Geometry check sheet. Reference: the model listing, model coordinates, mm. A direction names the side the tool comes from. Coordinates: 2 decimals unless noted, no trailing zeros. Loops run counter-clockwise (first coordinate to the right, second up) from the corner with the lowest first, then second, coordinate; pieces in that order, holes last. Notation, with made-up numbers: M -17,49.25 L 16,49.25 A25 cw 16,84.25 Z; hole C 52,67 d2. An arc over 180 degrees is marked long. Use CSV: the item, a comma, the result in double quotes.
```python
from build123d import *

# Parameters (mm, degrees)
EXTRUDE004_DEPTH                     = 10
SKETCH008_R                          = 3.1
EXTRUDE003_DEPTH                     = 10
EXTRUDE002_DEPTH                     = 2.65
EXTRUDE002_ONTO_SKETCH004_ROLL_ANGLE = 90
EXTRUDE001_DEPTH                     = 14
EXTRUDE_DEPTH                        = 30
EXTRUDE_ONTO_SKETCH_ROLL_ANGLE       = 90
FILLET_R                             = 10
POCKET_DEPTH                         = 20.001
SKETCH003_R                          = 1.55
POCKET001_DEPTH                      = 8
SKETCH005_W                          = 6
SKETCH005_H                          = 4
POCKET002_DEPTH                      = 9.5
SKETCH006_R                          = 4.1
POCKET003_DEPTH                      = 14.35
FILLET001_R                          = 2.5
FILLET002_R                          = 1
FILLET003_R                          = 2.5
FILLET004_R                          = 0.95
CHAMFER_SIZE2                        = 16
CHAMFER_SIZE                         = 6
CHAMFER001_SIZE                      = 5
SKETCH007_R                          = 1.55
POCKET004_DEPTH                      = 5.726
POCKET004_DEPTH_BACK                 = 6.476
FILLET005_R                          = 5
FILLET006_R                          = 0.65


with BuildPart() as extrude004:
    # Sketch009 → Extrude004 (new body)
    with BuildSketch(Plane(origin=(0.375, 0, 0), x_dir=(0, -1, 0), z_dir=(-1, 0, 0))):
        Polygon((-21.182001, 11.641407), (-23.86668, 10.091407), (-23.86668, 6.991407), (-21.182001, 5.441407), (-18.497322, 6.991407), (-18.497322, 10.091407), align=None)
    extrude(amount=-EXTRUDE004_DEPTH)


with BuildPart() as extrude004_1:
    # Extrude004 placement: moved
    add(extrude004.part.moved(Location((2, 0, 0))))


with BuildPart() as extrude003:
    # Sketch008 → Extrude003 (new body)
    with BuildSketch(Plane.YZ.offset(-0.375)):
        with Locations((21.182001, 8.541407)):
            Circle(SKETCH008_R)
    extrude(amount=-EXTRUDE003_DEPTH)


with BuildPart() as extrude003_1:
    # Extrude003 placement: moved
    add(extrude003.part.moved(Location((-2, 0, 0))))


with BuildPart() as extrude002:
    # Sketch004 as drawn → Extrude002 (new)
    with BuildSketch(Plane.XY):
        Polygon((0, -0.237971), (-2.825, -1.868985), (-2.825, -7), (2.825, -7), (2.825, -1.868985), align=None)
    extrude(amount=-EXTRUDE002_DEPTH)


with BuildPart() as extrude002_1:
    # Extrude002 onto Sketch004 roll: moved
    add(extrude002.part.rotate(Axis((0, 0, 0), (1, 0, 0)), EXTRUDE002_ONTO_SKETCH004_ROLL_ANGLE))


with BuildPart() as extrude002_2:
    # Extrude002 onto Sketch004 placement: moved
    add(extrude002_1.part.moved(Location((0, 4, 0))))


with BuildPart() as extrude002_3:
    # Extrude002 placement: moved
    add(extrude002_2.part.moved(Location((0, 3, 0))))


with BuildPart() as extrude001:
    # Sketch001 → Extrude001 (new body)
    with BuildSketch(Plane.YZ):
        Polygon((0, -7), (0, 0), (4, -3.5), (4, -7), align=None)
    extrude(amount=EXTRUDE001_DEPTH)


with BuildPart() as extrude001_1:
    # Extrude001 placement: moved
    add(extrude001.part.moved(Location((-7, 0, 0))))


with BuildPart() as fillet006:
    # Sketch as drawn → Extrude (new)
    with BuildSketch(Plane.XY):
        with BuildLine():
            Line((-6.1, -7), (6.1, -7))
            Line((6.1, -7), (6.1, 3.217039))
            Line((6.1, 3.217039), (4.375, 13))
            Line((4.375, 13), (0.375, 13))
            Line((0.375, 13), (0.375, 0.927025))
            ThreePointArc((-0.375, 0.927025), (0, -1), (0.375, 0.927025))
            Line((-0.375, 0.927025), (-0.375, 13))
            Line((-0.375, 13), (-4.375, 13))
            Line((-4.375, 13), (-6.1, 3.217039))
            Line((-6.1, 3.217039), (-6.1, -7))
        make_face()
    extrude(amount=-EXTRUDE_DEPTH)


with BuildPart() as fillet006_1:
    # Extrude onto Sketch roll: moved
    add(fillet006.part.rotate(Axis((0, 0, 0), (1, 0, 0)), EXTRUDE_ONTO_SKETCH_ROLL_ANGLE))


with BuildPart() as fillet006_2:
    # Extrude onto Sketch placement: moved
    add(fillet006_1.part)

    # Fillet
    fillet_edges = [fillet006_2.edges().sort_by_distance(p)[0] for p in [
        (-6.1, 15, 3.217039),
        (6.1, 15, 3.217039),
    ]]
    fillet(fillet_edges, radius=FILLET_R)

    # Sketch002 → Pocket (cut, through all)
    with BuildSketch(Plane(origin=(0, 0, -7), x_dir=(1, 0, 0), z_dir=(0, 0, -1))):
        with BuildLine():
            Line((-6.1, 0), (6.1, 0))
            ThreePointArc((-6.1, 0), (0, -1.366323), (6.1, 0))
        make_face()
    extrude(amount=-POCKET_DEPTH, mode=Mode.SUBTRACT)

    # Cut: cut Extrude001
    add(extrude001_1.part, mode=Mode.SUBTRACT)

    # Sketch003 → Pocket001 (cut, symmetric)
    with BuildSketch(Plane.XZ.offset(-4)):
        with Locations((0, -3.5)):
            Circle(SKETCH003_R)
    extrude(amount=POCKET001_DEPTH, both=True, mode=Mode.SUBTRACT)

    # Cut001: cut Extrude002
    add(extrude002_3.part, mode=Mode.SUBTRACT)

    # Sketch005 → Pocket002 (cut)
    with BuildSketch(Plane(origin=(0, 0, -7), x_dir=(1, 0, 0), z_dir=(0, 0, -1))):
        with Locations((0, -13.65)):
            Rectangle(SKETCH005_W, SKETCH005_H)
    extrude(amount=-POCKET002_DEPTH, mode=Mode.SUBTRACT)

    # Sketch006 → Pocket003 (cut)
    with BuildSketch(Plane(origin=(0, 30, 0), x_dir=(-1, 0, 0), z_dir=(0, 1, 0))):
        Circle(SKETCH006_R)
    extrude(amount=-POCKET003_DEPTH, mode=Mode.SUBTRACT)

    # Fillet001
    fillet001_edges = [fillet006_2.edges().sort_by_distance(p)[0] for p in [
        (-3, 13.65, 2.5),
        (3, 13.65, 2.5),
    ]]
    fillet(fillet001_edges, radius=FILLET001_R)

    # Fillet002
    fillet002_edges = [fillet006_2.edges().sort_by_distance(p)[0] for p in [
        (-3, 11.65, -3.5),
        (-2.267767, 11.65, 1.767767),
        (-0.4375, 11.65, 2.5),
        (3, 11.65, -3.5),
        (2.267767, 11.65, 1.767767),
        (0.4375, 11.65, 2.5),
    ]]
    fillet(fillet002_edges, radius=FILLET002_R)

    # Fillet003
    fillet003_edges = [fillet006_2.edges().sort_by_distance(p)[0] for p in [
        (0, 15.65, -4.1),
    ]]
    fillet(fillet003_edges, radius=FILLET003_R)

    # Fillet004
    fillet004_edges = [fillet006_2.edges().sort_by_distance(p)[0] for p in [
        (-3, 14.15, -7),
        (0, 15.65, -7),
        (-2.707107, 11.942893, -7),
        (0, 11.65, -7),
        (3, 14.15, -7),
        (2.707107, 11.942893, -7),
        (-2.825, 8.325, -7),
        (0, 7, -7),
        (0, 9.65, -7),
        (2.825, 8.325, -7),
    ]]
    fillet(fillet004_edges, radius=FILLET004_R)

    # Chamfer
    chamfer_edges = [fillet006_2.edges().sort_by_distance(p)[0] for p in [
        (2.399268, 1.16361, 13),
        (-2.399268, 1.16361, 13),
    ]]
    chamfer_side = fillet006_2.faces().sort_by_distance((0, 1.366323, -1.007857))[0]
    chamfer(chamfer_edges, length=CHAMFER_SIZE, length2=CHAMFER_SIZE2, reference=chamfer_side)

    # Chamfer001
    chamfer001_edges = [fillet006_2.edges().sort_by_distance(p)[0] for p in [
        (2.375, 30, 13),
        (-2.375, 30, 13),
    ]]
    chamfer(chamfer001_edges, length=CHAMFER001_SIZE)

    # Sketch007 → Pocket004 (cut, two sides)
    with BuildSketch(Plane.YZ.offset(-0.375)) as pocket004_sk:
        with Locations((21.182001, 8.541407)):
            Circle(SKETCH007_R)
    extrude(amount=-POCKET004_DEPTH, mode=Mode.SUBTRACT)
    extrude(pocket004_sk.sketch, amount=POCKET004_DEPTH_BACK, mode=Mode.SUBTRACT)

    # Fillet005
    fillet005_edges = [fillet006_2.edges().sort_by_distance(p)[0] for p in [
        (2.375, 25, 13),
        (2.380223, 17.272689, 13),
        (2.815817, 30, 8),
        (-2.815817, 30, 8),
        (-2.375, 25, 13),
        (-2.380223, 17.272689, 13),
    ]]
    fillet(fillet005_edges, radius=FILLET005_R)

    # Cut002: cut Extrude003
    add(extrude003_1.part, mode=Mode.SUBTRACT)

    # Cut003: cut Extrude004
    add(extrude004_1.part, mode=Mode.SUBTRACT)

    # Fillet006
    fillet006_edges = [fillet006_2.edges().sort_by_distance(p)[0] for p in [
        (0, 30, -7),
        (6.1, 17, -7),
        (-6.1, 17, -7),
        (0, 4, -7),
    ]]
    fillet(fillet006_edges, radius=FILLET006_R)


solid = fillet006_2.part
```
1. Section check A-A, the plane z = 6.5. Record the cut outline in (x, y) (1 decimal), plus the area to 3 significant figures.
The answers:
outline,"M -5.5,0.3 A14.3 cw -0.4,1.4 L -0.4,30 L -5.5,30 L -5.5,23.5 L -2.4,23.5 L -2.4,18.8 L -5.5,18.8 Z; M 0.4,1.4 A14.3 cw 5.5,0.3 L 5.5,19.3 L 2.4,19.3 L 2.4,23 L 5.5,23 L 5.5,30 L 0.4,30 Z"
area,"272 mm^2"
2. Section check C-C, the plane x = 0. Count the separate pieces of the cut face and the enclosed holes in it, plus the area to 3 significant figures.
The answers:
separate pieces,"5"
enclosed holes,"0"
area,"55.9 mm^2"
3. Gauge pin test, flat ends, axial feed: P1, Ø9.5, axis at y = 9, z = 8, coming from the -X side; P2, Ø5, axis at x = 5, y = 15.5, coming from the +Z side; P3, Ø0.9, axis at x = 2, z = -4.5, coming from the -Y side; P4, Ø1.6, axis at x = 0, z = 0, coming from the +Y side. Record the tip position at first contact, or that the pin passes through.
The answers:
P1,"x = -6.06"
P2,"z = 13"
P3,"y = 4"
P4,"through"
4. Thickness scan on line 1 (X direction, y = 7.5, z = -4.75) (3 decimals); line 2 (Z direction, x = -1.25, y = 22); line 3 (X direction, y = 22.25, z = 0). Record the ranges inside material, lowest first. Write a range as [from, to].
The answers:
line 1,"[-6.1, -2.825], [2.825, 6.1]"
line 2,"[-7, -3.9], [3.9, 7.22], [9.86, 13]"
line 3,"[-6.1, -4.1], [4.1, 6.1]"
5. Set-up check for faces 1 (the flat face through (-3, 15.65, 1)), 2 (the cylindrical face through (-2, 14, 2)), 3 (the flat face through (4, 18.497, 9)), 4 (the cylindrical face through (3.239, 8.357, -6.834)): record each of +Z, -Z, +X, -X, +Y, -Y from which the full face is reachable in a straight line by a thin tool's end or side.
The answers:
face 1,"+Y"
face 2,"-Z, +Y"
face 3,"+X"
face 4,"-Z"
6. Section check B-B, the plane y = 19. Record the cut outline in (x, z) (3 decimals), plus the area to 3 significant figures.
The answers:
outline,"M -6.1,-6.35 A0.65 ccw -5.45,-7 L 5.45,-7 A0.65 ccw 6.1,-6.35 L 6.1,2.342 A10 ccw 5.948,4.079 L 5.486,6.701 L 2.375,6.701 L 2.375,10.382 L 4.837,10.382 L 4.375,13 L 0.375,13 L 0.375,4.083 A4.1 cw long -0.375,4.083 L -0.375,13 L -4.375,13 L -4.773,10.743 L -2.375,10.743 L -2.375,6.339 L -5.549,6.339 L -5.948,4.079 A10 ccw -6.1,2.342 Z"
area,"145 mm^2"
7. Release check for a two-part mould opening along X. For faces 5 (the flat face through (4.018, 19.858, 6.206)), 6 (the flat face through (-5.325, 14.826, 7.611)), 7 (the flat face through (1.799, 8.306, -1.277)), 8 (the cylindrical face through (-1.87, 22.93, 3.65)) record: +X half, -X half, draft (parallel to the pull), parting line (faces both ways), or undercut.
The answers:
face 5,"draft"
face 6,"-X half"
face 7,"undercut"
face 8,"undercut"
